Input: part model. Units: mm. Frame: model coordinates. A direction names the side the tool comes from. Coordinates: 2 decimals unless noted, no trailing zeros. Order: outer loops, then holes, each group sorted by start corner. A loop starts at its lowest first (then second) coordinate and runs counter-clockwise, first axis right, second up. Notation, with made-up numbers: (-1.5, 80.5) -> (8.5, 80.5) arc R14 cw to (8.5, 94.5) -> close; hole circle Ø7 at (57.5, -12). An arc over 180 degrees is marked (long way). Write each question's results on one line, items separated by ' | '.
```python
from build123d import *

# Parameters (mm, degrees)
CROQUIS5_R              = 2
CORTAR_EXTRUIR1_DEPTH   = 6
CROQUIS6_R              = 23.5
CORTAR_EXTRUIR2_DEPTH   = 0.5
CROQUIS7_R              = 3.05
CROQUIS7_R_2            = 1.55
SALIENTE_EXTRUIR1_DEPTH = 9.5
CORTAR_EXTRUIR3_START   = -5.5
CROQUIS8_R              = 1.55
CORTAR_EXTRUIR3_DEPTH   = 5.5
REDONDEO1_R             = 2
REDONDEO2_R             = 2
CROQUIS9_R              = 23.5
CORTAR_EXTRUIR4_DEPTH   = 1


with BuildPart() as part:
    # Croquis3 → Revolución1 (revolve)
    with BuildSketch(Plane.XY):
        with BuildLine():
            Line((25, 0), (25, 3.742571384))
            ThreePointArc((25, 3.742571384), (21.675655898, 5.498663982), (18.228756555, 7))
            ThreePointArc((18.228756555, 7), (16.801415582, 9.620779584), (15, 12))
            Line((15, 12), (0, 12))
            Line((0, 12), (0, 0))
            Line((0, 0), (25, 0))
        make_face()
    revolve(axis=Axis((0, 0, 0), (0, 1, 0)))

    # Croquis4 → Cortar-Revolución1 (revolve, cut)
    with BuildSketch(Plane.XY):
        with BuildLine():
            Line((0, 1.5), (0, 10.5))
            Line((0, 10.5), (14.30686093, 10.5))
            ThreePointArc((14.30686093, 10.5), (15.877398251, 8.266411941), (17.102065618, 5.825983099))
            ThreePointArc((17.102065618, 5.825983099), (20.35484662, 4.463230038), (23.5, 2.867708066))
            Line((23.5, 2.867708066), (23.5, 1.5))
            Line((23.5, 1.5), (0, 1.5))
        make_face()
    revolve(axis=Axis((0, 10.5, 0), (0, 1, 0)), mode=Mode.SUBTRACT)

    # Croquis5 → Cortar-Extruir1 (cut)
    with BuildSketch(Plane(origin=(0, 12, 0), x_dir=(1, 0, 0), z_dir=(0, 1, 0))):
        with Locations(Location((0, 0, 0), (0, 0, 270))):
            Circle(CROQUIS5_R)
    extrude(amount=-CORTAR_EXTRUIR1_DEPTH, mode=Mode.SUBTRACT)

    # Croquis6 → Cortar-Extruir2 (cut)
    with BuildSketch(Plane.XZ):
        Circle(CROQUIS6_R)
    extrude(amount=-CORTAR_EXTRUIR2_DEPTH, mode=Mode.SUBTRACT)

    # Croquis7 → Saliente-Extruir1 (add)
    # profile 1 of 2: a face of its own
    with BuildSketch(Plane.XZ.offset(-10.5)):
        with Locations(Location((0, 10, 0), (0, 0, 180))):
            Circle(CROQUIS7_R)
        with Locations((0, 10)):
            Circle(CROQUIS7_R_2, mode=Mode.SUBTRACT)
    # profile 2 of 2: a face of its own
    with BuildSketch(Plane.XZ.offset(-10.5)):
        with Locations(Location((0, -10, 0), (0, 0, 180))):
            Circle(CROQUIS7_R)
        with Locations(Location((0, -10, 0), (0, 0, 90))):
            Circle(CROQUIS7_R_2, mode=Mode.SUBTRACT)
    extrude(amount=SALIENTE_EXTRUIR1_DEPTH)

    # Croquis8 → Cortar-Extruir3 (cut)
    with BuildSketch(Plane.XZ.offset(-10.5).offset(CORTAR_EXTRUIR3_START)):
        with Locations((0, -10)):
            Circle(CROQUIS8_R)
        with Locations((0, 10)):
            Circle(CROQUIS8_R)
    extrude(amount=CORTAR_EXTRUIR3_DEPTH, mode=Mode.SUBTRACT)

    # Redondeo1
    redondeo1_edges = [part.edges().sort_by_distance(p)[0] for p in [
        (-15, 12, 0),
    ]]
    fillet(redondeo1_edges, radius=REDONDEO1_R)

    # Redondeo2
    redondeo2_edges = [part.edges().sort_by_distance(p)[0] for p in [
        (-25, 3.742571384, 0),
    ]]
    fillet(redondeo2_edges, radius=REDONDEO2_R)

    # Croquis9 → Cortar-Extruir4 (cut)
    with BuildSketch(Plane.XZ.offset(-0.5)):
        Circle(CROQUIS9_R)
    extrude(amount=-CORTAR_EXTRUIR4_DEPTH, mode=Mode.SUBTRACT)


solid = part.part
```
(1) Pin query (flat end, axial travel): P1, Ø6.5, axis at x = -0.5, z = -10, coming from the -Y side; P2, Ø1.9, axis at x = 0, z = -10, coming from the +Y side; P3, Ø3, axis at x = -17.5, y = 5, coming from the +Z side; P4, Ø2, axis at y = 2, z = 5.5, coming from the +X side. Return the tip coordinate at first contact, or that it passes through.
Return value:
P1: y = 1.5 | P2: through | P3: z = 18.13 | P4: x = 24.59
(2) Reachability of faces 1 (the face through (-1.64, 6.06, 7.43)), 2 (the face through (-0.336, 6.823, 8.487)) from +Z, -Z, +X, -X, +Y, -Y: full face, straight path, thin tool, end or side. Return the list, or none.
Return value:
face 1: -Y | face 2: +Y, -Y
(3) Cut plane A-A, the plane y = 9. Return loops of the section in (x, z).
Return value:
outline: circle Ø34.37 at (0, 0); circle Ø6.1 at (0, -10); circle Ø6.1 at (0, 10); hole circle Ø30.83 at (0, 0); hole circle Ø3.1 at (0, -10); hole circle Ø3.1 at (0, 10)
(4) Mould query, pull axis Z, two halves, no side actions, for faces 3 (the face through (17, 0, 17)), 4 (the face through (23.846, 1.304, -7.509)), 5 (the face through (-1.64, 6.06, -12.57)). Classes: +Z half, -Z half, draft (parallel to the pull), parting line (faces both ways), or undercut.
Return value:
face 3: draft | face 4: parting line | face 5: undercut
(5) Line query: line 1 along Z through (x, y) = (0, 1); line 2 along X through (y, z) = (4.5, -10). Output: solid intervals per line, ascending. Write a range as from..to.
Return value:
line 1: -25..-23.5, 23.5..25 | line 2: -21.42..-17.64, -3.05..-1.55, 1.55..3.05, 17.64..21.42
(6) Cut plane B-B, the plane x = 0. Count the separate pieces of the cut face and the enclosed holes in it, plus the area to 3 significant figures.
Return value:
separate pieces: 4 | enclosed holes: 0 | area: 131 mm2
